Check sheet for the modelled part. Datum: model origin and axes. Units: mm. Face numbers are marked on the shaded views. A direction names the side the tool comes from. Round coordinates to 2 decimals unless told otherwise and drop trailing zeros. Write each loop counter-clockwise with the first axis right and the second up, starting at its lowest first coordinate (ties: lowest second). Pieces come first, ordered by that corner, then holes.
Item 1: Cross-section at A-A on y = -20.5. Enter the section's corners in (x, z).
Item 2: Release check for a two-part mould opening along X. For the marked faces 1, 2, 3 and 4 record: +X half, -X half, draft (parallel to the pull), parting line (faces both ways), or undercut.
Item 3: Go/stop test with flat-tipped pins: pin 1 Ø5 at (x, y) = (3, -10) entering from -Z (3 decimals); pin 2 Ø8 at (x, z) = (-16, 25.5) entering from -Y; pin 3 Ø3.5 at (x, z) = (-20, 21) entering from -Y; pin 4 Ø1 at (x, y) = (-7.5, 12) entering from -Z. Record where each tip stops, or that it passes through.
Item 4: Material ranges on line 1 (Y direction, x = 0, z = 29.85); line 2 (Y direction, x = -1, z = 34); line 3 (X direction, y = 0, z = 33.7), recorded low to high.
Item 5: Cross-section at C-C on x = 4.5. Count the separate pieces of the cut face and the enclosed holes in it, plus the area to 3 significant figures.
Item 6: Cross-section at B-B on z = 24. Enter the section's corners in (x, y).
Item 7: Tool access check on the marked faces 5, 6, 7 and 8. Record the directions out of +Z, -Z, +X, -X, +Y, -Y that give a thin tool (end or side, any length) a straight path to the whole face; none if there is none.
from build123d import *

# Parameters (mm, degrees)
SKETCH1_R               = 17
SKETCH1_R_2             = 16
BOSS_EXTRUDE1_DEPTH     = 37.3
BOSS_EXTRUDE3_START     = -3.175
SKETCH4_W               = 11.5
SKETCH4_H               = 11.5
BOSS_EXTRUDE3_DEPTH     = 3.175
SKETCH8_W               = 11.49524473
SKETCH8_H               = 29.000689646
SKETCH8_R               = 2.5875
BOSS_EXTRUDE4_DEPTH     = 5
CUT_EXTRUDE2_DEPTH      = 45.376683067
CUT_EXTRUDE2_DEPTH_BACK = 5
SKETCH7_R               = 5.15
SKETCH11_W              = 10.5
SKETCH11_H              = 6.75
CUT_EXTRUDE21_DEPTH     = 29
BOSS_EXTRUDE5_START     = -1.5
BOSS_EXTRUDE5_OUTLINE_R = 1.5
BOSS_EXTRUDE5_DEPTH     = 1.5
FILLET1_R               = 2.5
FILLET1_OF_MIRROR3_R    = 2.5
BOSS_EXTRUDE8_DEPTH     = 37.3
SKETCH15_8_W            = 5
SKETCH15_8_H            = 10
CUT_EXTRUDE22_DEPTH     = 37.3


# Read off the part's stored shape, not the designer's step: Boss-Extrude5
with BuildPart() as part:
    # Sketch1 → Boss-Extrude1 (new body)
    with BuildSketch(Plane.XY):
        with Locations(Location((0, 0, 0), (0, 0, 359.325928118))):
            Circle(SKETCH1_R)
        Circle(SKETCH1_R_2, mode=Mode.SUBTRACT)
    extrude(amount=BOSS_EXTRUDE1_DEPTH)

    # Sketch4 → Boss-Extrude3 (add)
    with BuildSketch(Plane.XY.offset(37.3).offset(BOSS_EXTRUDE3_START)):
        with BuildLine():
            ThreePointArc((-5.75, -14.931091722), (0, -16), (5.75, -14.931091722))
            Line((5.75, -14.931091722), (5.75, -5.75))
            Line((5.75, -5.75), (-5.75, -5.75))
            Line((-5.75, -5.75), (-5.75, -14.931091722))
        make_face()
        Rectangle(SKETCH4_W, SKETCH4_H)
        with BuildLine():
            ThreePointArc((5.75, 14.931091722), (0, 16), (-5.75, 14.931091722))
            Line((-5.75, 14.931091722), (-5.75, 5.75))
            Line((-5.75, 5.75), (5.75, 5.75))
            Line((5.75, 5.75), (5.75, 14.931091722))
        make_face()
    extrude(amount=BOSS_EXTRUDE3_DEPTH)

    # Sketch8 → Boss-Extrude4 (add)
    with BuildSketch(Plane.XY.offset(34.125)):
        Rectangle(SKETCH8_W, SKETCH8_H)
        Circle(SKETCH8_R, mode=Mode.SUBTRACT)
    extrude(amount=-BOSS_EXTRUDE4_DEPTH)

    # Sketch7 → Cut-Extrude2 (cut, two sides: drawn at the far end of the back side and taken through both)
    with BuildSketch(Plane.XY.offset(37.3).offset(-CUT_EXTRUDE2_DEPTH_BACK)):
        Circle(SKETCH7_R)
    extrude(amount=CUT_EXTRUDE2_DEPTH + CUT_EXTRUDE2_DEPTH_BACK, mode=Mode.SUBTRACT)

    # Sketch11 → Cut-Extrude21 (cut)
    with BuildSketch(Plane(origin=(0, 0, 37.3), x_dir=(-1, 0, 0), z_dir=(0, 0, -1))):
        with Locations((0, 9.025)):
            Rectangle(SKETCH11_W, SKETCH11_H)
    cut_extrude21 = extrude(amount=CUT_EXTRUDE21_DEPTH, mode=Mode.SUBTRACT)

    # Mirror1: Cut-Extrude21 across plane
    add(cut_extrude21.mirror(Plane.ZX), mode=Mode.SUBTRACT)

    # Boss-Extrude5 outline → Boss-Extrude5 (add)
    with BuildSketch(Plane(origin=(0, 0, 0), x_dir=(-1, 0, 0), z_dir=(0, 0, -1)).offset(BOSS_EXTRUDE5_START)):
        with BuildLine():
            ThreePointArc((-2.517959329, 16.812491809), (-0.018156734, 16.999990304), (2.482040671, 16.817832028))
            Line((2.482040671, 16.817832028), (2.482040671, 24))
            Line((2.482040671, 24), (-2.517959329, 24))
            Line((-2.517959329, 24), (-2.517959329, 16.812491809))
        make_face()
        with Locations((-0.017959329, 20.5)):
            Circle(BOSS_EXTRUDE5_OUTLINE_R, mode=Mode.SUBTRACT)
    boss_extrude5 = extrude(amount=BOSS_EXTRUDE5_DEPTH)

    # Fillet1
    fillet1_edges = [part.edges().sort_by_distance(p)[0] for p in [
        (2.517959329, 24, 0.75),
        (-2.482040671, 24, 0.75),
    ]]
    fillet(fillet1_edges, radius=FILLET1_R - 0.0001)  # a hair under: the kernel refuses the full size

    # Mirror3: Boss-Extrude5 across plane
    add(boss_extrude5.mirror(Plane.ZX))

    # Fillet1 of Mirror3
    fillet1_of_mirror3_edges = [part.edges().sort_by_distance(p)[0] for p in [
        (2.517959329, -24, 0.75),
        (-2.482040671, -24, 0.75),
    ]]
    fillet(fillet1_of_mirror3_edges, radius=FILLET1_OF_MIRROR3_R - 0.0001)  # a hair under: the kernel refuses the full size

    # Sketch15 → Boss-Extrude8 (add)
    with BuildSketch(Plane.XY):
        with BuildLine():
            Line((16.5, 5), (19, 5))
            Line((19, 5), (19, 6))
            Line((19, 6), (15.5, 6))
            Line((15.5, 6), (15.5, 3.968626967))
            ThreePointArc((15.5, 3.968626967), (15.874507866, 2), (16, 0))
            Line((16, 0), (16.5, 0))
            Line((16.5, 0), (16.5, 5))
        make_face()
        Polygon((21.5, 5), (21.5, 0), (22.5, 0), (22.5, 6), (19, 6), (19, 5), align=None)
        with BuildLine():
            Line((22.5, 0), (21.5, 0))
            Line((21.5, 0), (21.5, -5))
            Line((21.5, -5), (16.5, -5))
            Line((16.5, -5), (16.5, 0))
            Line((16.5, 0), (16, 0))
            ThreePointArc((16, 0), (15.874507866, -2), (15.5, -3.968626967))
            Line((15.5, -3.968626967), (15.5, -6))
            Line((15.5, -6), (22.5, -6))
            Line((22.5, -6), (22.5, 0))
        make_face()
    boss_extrude8 = extrude(amount=BOSS_EXTRUDE8_DEPTH)

    # Sketch15<8> → Cut-Extrude22 (cut)
    with BuildSketch(Plane.XY):
        with Locations((19, 0)):
            Rectangle(SKETCH15_8_W, SKETCH15_8_H)
    cut_extrude22 = extrude(amount=CUT_EXTRUDE22_DEPTH, mode=Mode.SUBTRACT)

    # Mirror4: Boss-Extrude8, Cut-Extrude22 across plane
    add(boss_extrude8.mirror(Plane(origin=(0, 0, 0), x_dir=(0, 0, 1), z_dir=(1, 0, 0))))
    add(cut_extrude22.mirror(Plane(origin=(0, 0, 0), x_dir=(0, 0, 1), z_dir=(1, 0, 0))), mode=Mode.SUBTRACT)


solid = part.part
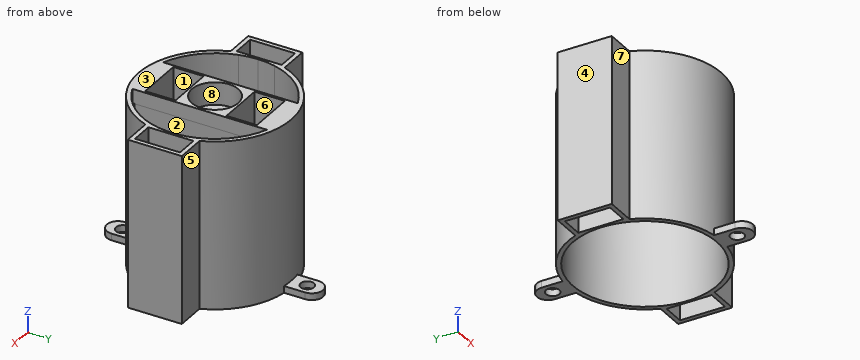
Response values:
1. outline: (-2.48, 0) - (-1.48, 0) - (-1.48, 1.5) - (-2.48, 1.5) - close; (1.52, 0) - (2.52, 0) - (2.52, 1.5) - (1.52, 1.5) - close
2. face 1: undercut
2. face 2: undercut
2. face 3: draft
2. face 4: -X half
3. pin 1: stops at z = 29.125
3. pin 2: stops at y = -12.04
3. pin 3: stops at y = -6
3. pin 4: passes through
4. line 1: y = -17 to -16, -14.5 to -12.4, -5.65 to -2.59, 2.59 to 5.65, 12.4 to 14.5, 16 to 17
4. line 2: y = -16.97 to -15.97, -14.5 to -12.4, -5.65 to -5.05, 5.05 to 5.65, 12.4 to 14.5, 15.97 to 16.97
4. line 3: x = -22.5 to -21.5, -16.5 to -16, -5.75 to -5.15, 5.15 to 5.75, 16 to 16.5, 21.5 to 22.5
5. separate pieces: 3
5. enclosed holes: 0
5. area: 185 mm2
6. outline: (-22.5, -6) - (-15.91, -6) arc R17 ccw to (15.91, -6) - (22.5, -6) - (22.5, 6) - (15.91, 6) arc R17 ccw to (-15.91, 6) - (-22.5, 6) - close; hole (-21.5, -5) - (-16.5, -5) - (-16.5, 5) - (-21.5, 5) - close; hole circle Ø32 at (0, 0); hole (16.5, -5) - (21.5, -5) - (21.5, 5) - (16.5, 5) - close
7. face 5: +Z, -Z, +X, +Y
7. face 6: +Z, -Z
7. face 7: +Z, -Z, -X, -Y
7. face 8: +Z
